```python
from build123d import *

# Parameters (mm, degrees)
BOSS_EXTRU_1_DEPTH      = 1.88
ESQUISSE2_R             = 3.95
BOSS_EXTRU_2_DEPTH      = 2.3
ESQUISSE3_R             = 2.4
ENL_V_MAT_EXTRU_1_DEPTH = 2.9
ESQUISSE4_R             = 1
ENL_V_MAT_EXTRU_2_DEPTH = 2.9


with BuildPart() as part:
    # Esquisse1 → Boss.-Extru.1 (new body)
    with BuildSketch(Plane(origin=(0, 0, 0), x_dir=(1, 0, 0), z_dir=(0, 1, 0))):
        with BuildLine():
            Line((-0.395, 3.930200377), (-15.245, 2.437719221))
            ThreePointArc((-15.245, 2.437719221), (-17.45, 0), (-15.245, -2.437719221))
            Line((-15.245, -2.437719221), (-0.395, -3.930200377))
            ThreePointArc((-0.395, -3.930200377), (0, -3.95), (0.395, -3.930200377))
            Line((0.395, -3.930200377), (15.245, -2.437719221))
            ThreePointArc((15.245, -2.437719221), (17.45, 0), (15.245, 2.437719221))
            Line((15.245, 2.437719221), (0.395, 3.930200377))
            ThreePointArc((0.395, 3.930200377), (0, 3.95), (-0.395, 3.930200377))
        make_face()
    extrude(amount=BOSS_EXTRU_1_DEPTH)

    # Esquisse2 → Boss.-Extru.2 (add)
    with BuildSketch(Plane(origin=(0, 1.88, 0), x_dir=(1, 0, 0), z_dir=(0, 1, 0))):
        with Locations(Location((0, 0, 0), (0, 0, 84.260829523))):
            Circle(ESQUISSE2_R)
    extrude(amount=BOSS_EXTRU_2_DEPTH)

    # Esquisse3 → Enlèv. mat.-Extru.1 (cut)
    with BuildSketch(Plane(origin=(0, 4.18, 0), x_dir=(1, 0, 0), z_dir=(0, 1, 0))):
        with Locations(Location((0, 0, 0), (0, 0, 270))):
            Circle(ESQUISSE3_R)
    extrude(amount=-ENL_V_MAT_EXTRU_1_DEPTH, mode=Mode.SUBTRACT)

    # Esquisse4 → Enlèv. mat.-Extru.2 (cut)
    with BuildSketch(Plane(origin=(0, 1.28, 0), x_dir=(1, 0, 0), z_dir=(0, 1, 0))):
        with Locations(Location((0, 0, 0), (0, 0, 270))):
            Circle(ESQUISSE4_R)
    extrude(amount=-ENL_V_MAT_EXTRU_2_DEPTH, mode=Mode.SUBTRACT)


solid = part.part
```
Read the model definition and answer for the solid it produces. Units are mm, in the model's axes. A direction names the side the tool comes from. Give positions to 0.01 mm unless a question says otherwise; leave off trailing zeros. Order: outer loops, then holes, each group sorted by start corner. A loop starts at its lowest first (then second) coordinate and runs counter-clockwise, first axis right, second up. Notation, with made-up numbers: (82.25, 88) -> (111.25, 88) arc R33 ccw to (111.25, 123) -> close; hole circle Ø4 at (63, 17.25). An arc over 180 degrees is marked (long way). One line per item, written item: value. Start each with the question number.
(1) The part is cut by section B-B (z = 0). Determine the outline of the cut face in (x, y), and give its area (3 significant figures).
(2) Straight lines are drawn through the part: L1, parallel to X at y = 2.35, z = 0; L2, parallel to X at y = 0.9, z = 0; L3, parallel to Y at x = 4, z = -2.5. For each, find the intervals that lie inside material, in ascending order.
(3) The part is cut by section C-C (y = 0.65). Determine the outline of the cut face in (x, z) (3 decimals), and give its area (3 significant figures).
(4) Flat-ended cylindrical pins translate along their axes: P1, Ø1, axis at y = 0.5, z = -1.5, coming from the +X side; P2, Ø2.5, axis at x = 12.5, z = -0.5, coming from the +Y side; P3, Ø1, axis at y = 3, z = 2, coming from the +X side; P4, Ø1.2, axis at x = 0, z = 0, coming from the +Y side. Find the tip coordinate at first contact, or state that the pin passes through.
(5) A tool of negligible diameter and unlimited length cuts with its end or side. For faces 4 (the flat face through (7.716, 0.927, 3.194)), 5 (the cylindrical face through (2.024, 2.75, 1.29)), from which of +Z, -Z, +X, -X, +Y, -Y can it reach the whole face along a straight path? Write none if from no direction.
(6) The part is cut by section A-A (x = 0). Determine the outline of the cut face in (y, z).
(7) The part is cut by section D-D (z = 3.5). Determine the outline of the cut face in (x, y), and give its area (3 significant figures).
(8) For a pull along Z with two mould halves and no side action, classify faces 1 (the cylindrical face through (-1, 1, 0)), 2 (the flat face through (-7.924, 0.927, 3.174)), 3 (the flat face through (0, 0, 2)) as released by +Z, released by -Z, zero draft, split by the parting line, or undercut.
Taken from the geometry:
1. outline: (-17.45, 0) -> (-1, 0) -> (-1, 1.28) -> (-2.4, 1.28) -> (-2.4, 4.18) -> (-3.95, 4.18) -> (-3.95, 1.88) -> (-17.45, 1.88) -> close; (1, 0) -> (17.45, 0) -> (17.45, 1.88) -> (3.95, 1.88) -> (3.95, 4.18) -> (2.4, 4.18) -> (2.4, 1.28) -> (1, 1.28) -> close
1. area: 67.3 mm^2
2. L1: -3.95 to -2.4, 2.4 to 3.95
2. L2: -17.45 to -1, 1 to 17.45
2. L3: 0 to 1.88
3. outline: (-15.245, -2.438) -> (-0.395, -3.93) arc R3.95 ccw to (0.395, -3.93) -> (15.245, -2.438) arc R2.45 ccw to (15.245, 2.438) -> (0.395, 3.93) arc R3.95 ccw to (-0.395, 3.93) -> (-15.245, 2.438) arc R2.45 ccw to start; hole circle Ø2 at (0, 0)
3. area: 209 mm^2
4. P1: x = 17.24
4. P2: y = 1.88
4. P3: x = 3.65
4. P4: through
5. face 4: +Z, +X, +Y, -Y
5. face 5: +Y
6. outline: (0, -3.95) -> (4.18, -3.95) -> (4.18, -2.4) -> (1.28, -2.4) -> (1.28, -1) -> (0, -1) -> close; (0, 1) -> (1.28, 1) -> (1.28, 2.4) -> (4.18, 2.4) -> (4.18, 3.95) -> (0, 3.95) -> close
7. outline: (-4.68, 0) -> (4.68, 0) -> (4.68, 1.88) -> (1.83, 1.88) -> (1.83, 4.18) -> (-1.83, 4.18) -> (-1.83, 1.88) -> (-4.68, 1.88) -> close
7. area: 26.0 mm^2
8. face 1: undercut
8. face 2: released by +Z
8. face 3: zero draft
